from build123d import *

# Parameters (mm, degrees)
SKETCH_1_W          = 40
SKETCH_1_H          = 100
EXTRUDE_1_DEPTH     = 5.5
SKETCH_2_W          = 5.5
SKETCH_2_H          = 10
CUT_EXTRUDE_1_DEPTH = 55.13178364
SKETCH_3_W          = 10
SKETCH_3_H          = 5.5
CUT_EXTRUDE_2_DEPTH = 55.13178364


with BuildPart() as part:
    # ｽｹｯﾁ1 → ﾎﾞｽ - 押し出し1 (new body)
    with BuildSketch(Plane.XY):
        Rectangle(SKETCH_1_W, SKETCH_1_H)
    extrude(amount=EXTRUDE_1_DEPTH)

    # ｽｹｯﾁ2 → ｶｯﾄ - 押し出し1 (cut, through all)
    with BuildSketch(Plane.XY.offset(5.5)):
        with Locations((-17.25, -45)):
            Rectangle(SKETCH_2_W, SKETCH_2_H)
        with Locations((17.25, -35)):
            Rectangle(SKETCH_2_W, SKETCH_2_H)
        with Locations((-17.25, -25)):
            Rectangle(SKETCH_2_W, SKETCH_2_H)
        with Locations((17.25, -15)):
            Rectangle(SKETCH_2_W, SKETCH_2_H)
        with Locations((-17.25, -5)):
            Rectangle(SKETCH_2_W, SKETCH_2_H)
        with Locations((17.25, 5)):
            Rectangle(SKETCH_2_W, SKETCH_2_H)
        with Locations((-17.25, 15)):
            Rectangle(SKETCH_2_W, SKETCH_2_H)
        with Locations((17.25, 25)):
            Rectangle(SKETCH_2_W, SKETCH_2_H)
        with Locations((-17.25, 35)):
            Rectangle(SKETCH_2_W, SKETCH_2_H)
        with Locations((17.25, 45)):
            Rectangle(SKETCH_2_W, SKETCH_2_H)
    extrude(amount=-CUT_EXTRUDE_1_DEPTH, mode=Mode.SUBTRACT)

    # ｽｹｯﾁ3 → ｶｯﾄ - 押し出し2 (cut, through all)
    with BuildSketch(Plane.XY.offset(5.5)):
        with Locations((0, 47.25)):
            Rectangle(SKETCH_3_W, SKETCH_3_H)
    extrude(amount=-CUT_EXTRUDE_2_DEPTH, mode=Mode.SUBTRACT)


solid = part.part
Part model, mm, in its own coordinate system. A direction names the side the tool comes from. Round coordinates to 2 decimals unless told otherwise and drop trailing zeros. Write each loop counter-clockwise with the first axis right and the second up, starting at its lowest first coordinate (ties: lowest second). Pieces come first, ordered by that corner, then holes. Notation, with made-up numbers: M 8.25,-9.5 L 61.25,-9.5 A35 cw 61.25,23.5 Z; hole C -17.75,62.5 d11. An arc over 180 degrees is marked long. Return JSON: item names as keys, results as strings. Group by question number.
(1) Drill centre lines: probe 1 along Y at (x, z) = (-15, 3.25); probe 2 along Y at (x, z) = (16.5, 2.35); probe 3 along X at (y, z) = (-24.5, 3.8). Where is each one in solid material? Low to high.
(2) Saw through at B-B on x = 0.5. Write the cut outline in (y, z), then the cut area to 3 significant figures.
(3) Pin check, flat tips, straight feed: pin 1 Ø3 at (x, z) = (18, 4) entering from +Y; pin 2 Ø3 at (x, z) = (-17.5, 2) entering from -Y; pin 3 Ø1.6 at (y, z) = (-3, 2) entering from -X. Stop position of each tip, or through.
(4) Saw through at C-C on y = 7.5. Write the cut outline in (x, z).
(5) Two-plate mould, pull along Y, no slides. Class faces 5 (the face through (0, 1, 5.5)), 6 (the face through (-17, 10, 3)), 7 (the face through (17, 40, 3)): +Y half, -Y half, draft (parallel to the pull), parting line (faces both ways), or undercut.
(6) Which spindle directions (+Z, -Z, +X, -X, +Y, -Y) get a long thin tool onto all of the face, cutting with end or side? Do faces 1 (the face through (-17, -10, 3)), 2 (the face through (14.5, 45, 3)), 3 (the face through (17, 0, 3)), 4 (the face through (-17, -40, 3)). Say none if no direction does.
(7) Saw through at A-A on x = 17.5. Write the cut outline in (y, z), then the cut area to 3 significant figures.
Returned:
{
 "1": {"probe 1": "-40 to -30, -20 to -10, 0 to 10, 20 to 30, 40 to 50", "probe 2": "-50 to -40, -30 to -20, -10 to 0, 10 to 20, 30 to 40", "probe 3": "-14.5 to 20"},
 "2": {"outline": "M -50,0 L 44.5,0 L 44.5,5.5 L -50,5.5 Z", "area": "520 mm²"},
 "3": {"pin 1": "y = 40", "pin 2": "y = -40", "pin 3": "x = -14.5"},
 "4": {"outline": "M -20,0 L 14.5,0 L 14.5,5.5 L -20,5.5 Z"},
 "5": {"face 5": "draft", "face 6": "undercut", "face 7": "+Y half"},
 "6": {"face 1": "+Z, -Z, -X", "face 2": "+Z, -Z, +X, +Y", "face 3": "+Z, -Z, +X", "face 4": "+Z, -Z, -X, -Y"},
 "7": {"outline": "M -50,0 L -40,0 L -40,5.5 L -50,5.5 Z; M -30,0 L -20,0 L -20,5.5 L -30,5.5 Z; M -10,0 L 0,0 L 0,5.5 L -10,5.5 Z; M 10,0 L 20,0 L 20,5.5 L 10,5.5 Z; M 30,0 L 40,0 L 40,5.5 L 30,5.5 Z", "area": "275 mm²"}
}
